Autodesk Inventor part; units mm, degrees
ref_plane "YZ Plane" through (0, 0, 0) normal (1, 0, 0) x (0, 1, 0)
ref_plane "XY Plane" through (0, 0, 0) normal (0, 0, 1) x (1, 0, 0)
sketch "Sketch1" plane through (0, 0, 0) normal (0, 1, 0) x (-1, 0, 0)
  line L0 (-60, -60) -> (60, -60)
  line L1 (60, -60) -> (60, 60)
  line L2 (60, 60) -> (-60, 60)
  line L3 (-60, 60) -> (-60, -60)
  line L4 (-60, -60) -> (60, 60) construction
  line L5 (60, -60) -> (-60, 60) construction
  line L6 (-29, -29) -> (29, 29) construction
  line L7 (28, -28) -> (-28, 28) construction
  line L8 (-36.5, -36.5) -> (36.5, 36.5) construction
  line L9 (36.5, -36.5) -> (-36.5, 36.5) construction
  line L10 (-39, -39) -> (39, 39) construction
  line L11 (33.9, -33.9) -> (-33.9, 33.9) construction
  line L12 (-24.8, -24.8) -> (24.8, 24.8) construction
  line L13 (39.8, -39.8) -> (-39.8, 39.8) construction
  line L14 (-39, -39) -> (39, -39)
  line L15 (39, -39) -> (39, 39)
  line L16 (39, 39) -> (-39, 39)
  line L17 (-39, 39) -> (-39, -39)
  line L18 (-39, -39) -> (39, 39) construction
  line L19 (39, -39) -> (-39, 39) construction
  line L20 (-29, -29) -> (29, -29)
  line L21 (29, -29) -> (29, 29)
  line L22 (29, 29) -> (-29, 29)
  line L23 (-29, 29) -> (-29, -29)
  line L24 (-29, -29) -> (29, 29) construction
  line L25 (29, -29) -> (-29, 29) construction
  point P0 (0, 0)
  dimension "d0" = 120
  dimension "d1" = 120
  dimension "d13" = 78
  dimension "d14" = 78
  dimension "Largo_PaP" = 58
  dimension "Ancho_PaP" = 58
extrude "Extrusion1" add sketch "Sketch1" along normal blind 22 contours L3 L2 L1 L0
extrude "Extrusion2" add sketch "Sketch1" along normal blind 62 contours L17 L16 L15 L14
sketch "Sketch2" plane through (0, 22, 0) normal (0, 1, 0) x (1, 0, 0)
  line L0 (-60, 60) -> (-60, -60)
  line L1 (60, -60) -> (60, 60)
  line L2 (-60, -60) -> (60, -60)
  line L3 (60, 60) -> (-60, 60)
  line L4 (50, 50) -> (-50, 50)
  line L5 (-50, 50) -> (-50, -50)
  line L6 (-50, -50) -> (50, -50)
  line L7 (50, -50) -> (50, 50)
  line L8 (50, 50) -> (-50, -50) construction
  line L9 (-50, 50) -> (50, -50) construction
  point P0 (50, 0)
  point P1 (0, 50)
  point P2 (-50, 0)
  dimension "d82" = 100
  dimension "d83" = 100
hole "Hole1" at (-50, 22, 50) at (50, 22, 50) at (50, 22, -50) at (0, 22, -50) at (-50, 22, -50) at (-50, 22, 0) at (50, 22, 0) direction (0, -1, 0) diameter 6.1 end through all
sketch "Sketch3" plane through (0, 62, 0) normal (0, 1, 0) x (1, 0, 0)
  line L0 (29, -29) -> (-29, -29)
  line L1 (29, 29) -> (-29, 29)
  line L2 (-29, 29) -> (-29, -29)
  line L3 (-29, -29) -> (29, -29)
  line L4 (29, -29) -> (29, 29)
  line L5 (29, 29) -> (-29, -29) construction
  line L6 (-29, 29) -> (29, -29) construction
  line L7 (14, -14) -> (-14, 14) construction
  line L8 (-14, -14) -> (14, 14) construction
  line L9 (19, -19) -> (-19, 19) construction
  line L10 (-19, -19) -> (19, 19) construction
  circle A0 centre (0, 0) radius 19.15
  dimension "d56" = 38.3
extrude "Extrusion3" add sketch "Sketch3" against normal blind 8
fillet "Fillet1" radius 2 8 edges at (0, 22, 60) (-60, 22, 0) (60, 22, 0) (0, 22, -60) (60, 11, 60) (-60, 11, 60) (60, 11, -60) (-60, 11, -60)
fillet "Fillet2" radius 1 8 edges at (0, 62, 39) (39, 62, 0) (0, 62, -39) (-39, 62, 0) (-39, 42, -39) (39, 42, -39) (-39, 42, 39) (39, 42, 39)
sketch "Sketch4" plane through (0, 62, 0) normal (0, 1, 0) x (1, 0, 0)
  line L0 (39, -38) -> (39, 38)
  line L1 (-38, -39) -> (38, -39)
  line L2 (0, -10.7148) -> (0, 11.656) construction
  line L3 (7.4793, 0) -> (-11.1938, 0) construction
  line L4 (28, 28) -> (-28, 28)
  line L5 (-28, 28) -> (-28, -28)
  line L6 (-28, -28) -> (28, -28)
  line L7 (28, -28) -> (28, 28)
  line L8 (28, 28) -> (-28, -28) construction
  line L9 (-28, 28) -> (28, -28) construction
  point P0 (0, 0)
  point P1 (23.5, -23.5)
  point P2 (-23.5, -23.5)
  point P3 (23.5, 23.5)
  point P4 (-23.5, 23.5)
  dimension "d53" = 56
  dimension "d54" = 56
  dimension "d57" = 47
  dimension "d58" = 47
hole "Hole2" at (-23.5, 62, 23.5) at (23.5, 62, 23.5) at (23.5, 62, -23.5) at (-23.5, 62, -23.5) direction (0, -1, 0) diameter 5.5 end through all
sketch "Sketch6" plane through (0, 62, 0) normal (0, 1, 0) x (1, 0, 0)
  circle A0 centre (0, 0) radius 19.15
  circle A1 centre (0, 0) radius 10
  dimension "d59" = 20
  dimension "d60" = 38.3
extrude "Extrusion4" add sketch "Sketch6" against normal blind 5
sketch "Sketch12" plane through (0, 62, 0) normal (0, 1, 0) x (1, 0, 0)
  circle A0 centre (0, 0) radius 26.15
  circle A1 centre (0, 0) radius 10
  dimension "d85" = 52.3
extrude "Extrusion9" add sketch "Sketch12" along normal blind 28
sketch "Sketch13" plane through (0, 90, 0) normal (0, 1, 0) x (1, 0, 0)
  circle A0 centre (0, 0) radius 4.5
  circle A1 centre (0, 0) radius 10
  circle A2 centre (0, 0) radius 26.15
  dimension "d88" = 9
extrude "Extrusion10" add sketch "Sketch13" along normal blind 20 contours A1 | A2
sketch "Sketch9" plane through (-58, 0, 60) normal (0, 0, 1) x (1, 0, 0)
  line L0 (0, 0) -> (0, 20) construction
  line L1 (0, 0) -> (116, 0) construction
  line L2 (0, 0) -> (116, 0) construction
  line L3 (64.5, -14) -> (51.5, -14)
  line L4 (51.5, -14) -> (51.5, 14)
  line L5 (51.5, 14) -> (64.5, 14)
  line L6 (64.5, 14) -> (64.5, -14)
  line L7 (64.5, -14) -> (51.5, 14) construction
  line L8 (51.5, -14) -> (64.5, 14) construction
  point P0 (58, 0)
  dimension "d77" = 13
  dimension "d78" = 28
extrude "Extrusion8" cut sketch "Sketch9" against normal up to surface (31 mm away)
sketch "Sketch14" plane through (0, 110, 0) normal (0, 1, 0) x (1, 0, 0)
  circle A0 centre (0, 0) radius 10.9
  circle A1 centre (0, 0) radius 26.15
  dimension "d91" = 21.8
extrude "Extrusion11" add sketch "Sketch14" along normal blind 10
ref_plane "Work Plane3" through (0, 81.25, 0) normal (0, 1, 0) x (-1, 0, 0)
sketch "Sketch15" plane through (0, 120, 0) normal (0, 1, 0) x (1, 0, 0)
  point P0 (0, 0)
equation "\"Largo_PaP\" = Ancho_PaP"
properties part number "Eslabón1"
Part model, mm, in its own coordinate system. A direction names the side the tool comes from. Give positions to 0.01 mm unless a question says otherwise; leave off trailing zeros. Order: outer loops, then holes, each group sorted by start corner. A loop starts at its lowest first (then second) coordinate and runs counter-clockwise, first axis right, second up. Notation, with made-up numbers: (-4.5, 43) - (8.5, 43) arc R20 ccw to (8.5, 48) - close; hole circle Ø11 at (16.25, 60.25). An arc over 180 degrees is marked (long way). Use one line per item in the form item = value.
Item 1: Two-plate mould, pull along X, no slides. Class faces 1 (the face through (-0.4, 120, 11.3)), 2 (the face through (-39, 41, -1)), 3 (the face through (0, 27, 29)): released by +X, released by -X, zero draft, split by the parting line, or undercut.
Solution:
face_1 = zero draft
face_2 = released by -X
face_3 = undercut
Item 2: Slice it at A-A on z = 50. Give the cut face in (x, y), and give its area (3 significant figures).
Solution:
outline = (-60, 0) - (-53.05, 0) - (-53.05, 22) - (-58, 22) arc R2 ccw to (-60, 20) - close; (-46.95, 0) - (-6.5, 0) - (-6.5, 14) - (6.5, 14) - (6.5, 0) - (46.95, 0) - (46.95, 22) - (-46.95, 22) - close; (53.05, 0) - (60, 0) - (60, 20) arc R2 ccw to (58, 22) - (53.05, 22) - close
area = 2,190 mm2
Item 3: Slice it at C-C on z = -50. Give the cut face in (x, y).
Solution:
outline = (-60, 0) - (-53.05, 0) - (-53.05, 22) - (-58, 22) arc R2 ccw to (-60, 20) - close; (-46.95, 0) - (-3.05, 0) - (-3.05, 22) - (-46.95, 22) - close; (3.05, 0) - (46.95, 0) - (46.95, 22) - (3.05, 22) - close; (53.05, 0) - (60, 0) - (60, 20) arc R2 ccw to (58, 22) - (53.05, 22) - close
Item 4: Which spindle directions (+Z, -Z, +X, -X, +Y, -Y) get a long thin tool onto all of the face, cutting with end or side? Do faces 4 (the face through (0, 54, -20)), 5 (the face through (-6.5, 7, 45)), 6 (the face through (-47.023, 10.846, -0.661)), 7 (the face through (0, 110, 5)), 8 (the face through (41, 0, 1)). Say none if no direction does.
Solution:
face_4 = -Y
face_5 = +Z, -Y
face_6 = +Y, -Y
face_7 = +Y
face_8 = +Z, -Z, +X, -X, -Y
Item 5: Pin check, flat tips, straight feed: pin 1 Ø8 at (x, z) = (-50, -50) entering from +Y; pin 2 Ø9 at (x, z) = (-23.5, -23.5) entering from -Y; pin 3 Ø3.5 at (x, z) = (0, -50) entering from +Y; pin 4 Ø17.5 at (x, z) = (-7, 3) entering from -Y. Stop position of each tip, or through.
Solution:
pin_1 = 22
pin_2 = 54
pin_3 = through
pin_4 = 57
Item 6: Slice it at B-B on x = -31. Give the cut face in (y, z), and give its area (3 significant figures).
Solution:
outline = (0, -60) - (20, -60) arc R2 ccw to (22, -58) - (22, -39) - (61, -39) arc R1 ccw to (62, -38) - (62, 38) arc R1 ccw to (61, 39) - (22, 39) - (22, 58) arc R2 ccw to (20, 60) - (0, 60) - close
area = 5,760 mm2
Item 7: Probe probe 1 along X at (y, z) = (10, -50); probe 2 along X at (y, z) = (59, -23.5). List the from-to ranges inside material, lowest first. Write a range as from..to.
Solution:
probe_1 = -60..-53.05, -46.95..-3.05, 3.05..46.95, 53.05..60
probe_2 = -39..-26.25, -20.75..20.75, 26.25..39
Item 8: Slice it at D-D on y = 31.5. Give the cut face in (x, z), and give its area (3 significant figures).
Solution:
outline = (-39, -38) arc R1 ccw to (-38, -39) - (38, -39) arc R1 ccw to (39, -38) - (39, 38) arc R1 ccw to (38, 39) - (-38, 39) arc R1 ccw to (-39, 38) - close; hole (-29, -29) - (29, -29) - (29, 29) - (-29, 29) - close
area = 2,720 mm2
